Can you work these out from the model? Positions are in its coordinate system, mm. A direction names the side the tool comes from. Give positions to 0.01 mm unless a question says otherwise; leave off trailing zeros. Order: outer loops, then holes, each group sorted by start corner. A loop starts at its lowest first (then second) coordinate and runs counter-clockwise, first axis right, second up. Notation, with made-up numbers: M 19,-22 L 24,-22 A15 ccw 24,-7 Z; hole C -2.5,76 d6. An arc over 180 degrees is marked long. Answer as a JSON object with one key per item and string values.
```python
from build123d import *

# Parameters (mm, degrees)
SKETCH1_W           = 52
SKETCH1_H           = 24
SKETCH1_R           = 8.25
BOSS_EXTRUDE1_DEPTH = 12
SKETCH2_R           = 1
CUT_EXTRUDE1_DEPTH  = 32.048349393
SKETCH3_R           = 1.75
CUT_EXTRUDE2_DEPTH  = 1
FILLET1_R           = 2.5
CUT_EXTRUDE3_DEPTH  = 5
FILLET2_R           = 0.5
SKETCH6_W           = 10
SKETCH6_H           = 10
SKETCH6_R           = 2
BOSS_EXTRUDE2_DEPTH = 5
FILLET3_R           = 4.6
FILLET4_R           = 3


with BuildPart() as part:
    # Sketch1 → Boss-Extrude1 (new body)
    with BuildSketch(Plane(origin=(0, 0, 0), x_dir=(1, 0, 0), z_dir=(0, 1, 0))):
        Rectangle(SKETCH1_W, SKETCH1_H)
        with Locations(Location((12.75, 0, 0), (0, 0, 270))):
            Circle(SKETCH1_R, mode=Mode.SUBTRACT)
        with Locations(Location((-12.75, 0, 0), (0, 0, 270))):
            Circle(SKETCH1_R, mode=Mode.SUBTRACT)
    extrude(amount=BOSS_EXTRUDE1_DEPTH)

    # Sketch2 → Cut-Extrude1 (cut, through all)
    with BuildSketch(Plane(origin=(0, 12, 0), x_dir=(1, 0, 0), z_dir=(0, 1, 0))):
        with Locations(Location((-21.35, 8.85, 0), (0, 0, 270))):
            Circle(SKETCH2_R)
        with Locations(Location((21.35, 8.85, 0), (0, 0, 270))):
            Circle(SKETCH2_R)
        with Locations(Location((21.35, -8.85, 0), (0, 0, 270))):
            Circle(SKETCH2_R)
        with Locations(Location((-21.35, -8.85, 0), (0, 0, 270))):
            Circle(SKETCH2_R)
    extrude(amount=-CUT_EXTRUDE1_DEPTH, mode=Mode.SUBTRACT)

    # Sketch3 → Cut-Extrude2 (cut)
    with BuildSketch(Plane(origin=(0, 12, 0), x_dir=(1, 0, 0), z_dir=(0, 1, 0))):
        with Locations(Location((-21.35, 8.85, 0), (0, 0, 270))):
            Circle(SKETCH3_R)
        with Locations(Location((21.35, 8.85, 0), (0, 0, 270))):
            Circle(SKETCH3_R)
        with Locations(Location((21.35, -8.85, 0), (0, 0, 270))):
            Circle(SKETCH3_R)
        with Locations(Location((-21.35, -8.85, 0), (0, 0, 270))):
            Circle(SKETCH3_R)
    extrude(amount=-CUT_EXTRUDE2_DEPTH, mode=Mode.SUBTRACT)

    # Fillet1
    fillet1_edges = [part.edges().sort_by_distance(p)[0] for p in [
        (26, 6, 12),
        (-26, 6, 12),
        (-26, 6, -12),
        (26, 6, -12),
    ]]
    fillet(fillet1_edges, radius=FILLET1_R)

    # Sketch4 → Cut-Extrude3 (cut)
    with BuildSketch(Plane.XZ):
        Polygon((-6, -5), (-6, -12), (6, -12), (6, -5), (0, -5), align=None)
    extrude(amount=-CUT_EXTRUDE3_DEPTH, mode=Mode.SUBTRACT)

    # Fillet2
    fillet2_edges = [part.edges().sort_by_distance(p)[0] for p in [
        (0, 5, -12),
        (6, 2.5, -12),
        (-6, 2.5, -12),
        (-6, 2.5, -5),
        (6, 5, -8.5),
        (6, 2.5, -5),
        (-6, 5, -8.5),
        (0, 5, -5),
    ]]
    fillet(fillet2_edges, radius=FILLET2_R)

    # Sketch6 → Boss-Extrude2 (add)
    # profile 1 of 2: a face of its own
    with BuildSketch(Plane(origin=(0, 12, 0), x_dir=(1, 0, 0), z_dir=(0, 1, 0))):
        with Locations((-31, 0)):
            Rectangle(SKETCH6_W, SKETCH6_H)
        with Locations(Location((-31, 0, 0), (0, 0, 270))):
            Circle(SKETCH6_R, mode=Mode.SUBTRACT)
    # profile 2 of 2: a face of its own
    with BuildSketch(Plane(origin=(0, 12, 0), x_dir=(1, 0, 0), z_dir=(0, 1, 0))):
        with Locations((31, 0)):
            Rectangle(SKETCH6_W, SKETCH6_H)
        with Locations(Location((31, 0, 0), (0, 0, 90))):
            Circle(SKETCH6_R, mode=Mode.SUBTRACT)
    extrude(amount=-BOSS_EXTRUDE2_DEPTH)

    # Fillet3
    # the kernel refuses this fillet: 4.6 mm, written as the material it adds along each edge
    with BuildSketch(Plane(origin=(26, 12, 5), x_dir=(-5.467859312132584e-05, 0, 0.9999999985051258), z_dir=(0, -1, 0)), Plane(origin=(-26, 12, -5), x_dir=(5.467859312132586e-05, 0, -0.9999999985051258), z_dir=(0, -1, 0))) as fillet3_piece_1:
        with BuildLine():
            CenterArc((4.59974851, -4.599547254), FILLET3_R, 90.80387664, 89.192990507)
            Line((-0.000251483, -4.599295733), (-0.460251482, -4.599270581))
            Line((-0.460251482, -4.599270581), (-0.459999999, 2.5152e-05))
            Line((-0.459999999, 2.5152e-05), (2.5152e-05, 0.459999999))
            ThreePointArc((2.5152e-05, 0.459999999), (4.500025145, 0.459753946), (4.528757551, 0.459954725))
            Line((4.528757551, 0.459954725), (4.535211274, 0))
        make_face()
    extrude(amount=5)
    with BuildSketch(Plane(origin=(-26, 12, 5), x_dir=(5.467859312289258e-05, 0, 0.9999999985051258), z_dir=(0, -1, 0)), Plane(origin=(26, 12, -5), x_dir=(-5.467859312132581e-05, 0, -0.9999999985051258), z_dir=(0, -1, 0))) as fillet3_piece_2:
        with BuildLine():
            CenterArc((4.59974851, 4.599547254), FILLET3_R, 180.003132853, 89.192990507)
            Line((-0.000251483, 4.599295733), (-0.460251482, 4.599270581))
            Line((-0.460251482, 4.599270581), (-0.459999999, -2.5152e-05))
            Line((-0.459999999, -2.5152e-05), (2.5152e-05, -0.459999999))
            ThreePointArc((2.5152e-05, -0.459999999), (4.500025145, -0.459753946), (4.528757551, -0.459954725))
            Line((4.528757551, -0.459954725), (4.535211274, 0))
        make_face()
    extrude(amount=5)

    # Fillet4
    fillet4_edges = [part.edges().sort_by_distance(p)[0] for p in [
        (-36, 9.5, 5),
        (-36, 9.5, -5),
        (36, 9.5, -5),
        (36, 9.5, 5),
    ]]
    fillet(fillet4_edges, radius=FILLET4_R)


solid = part.part
```
1) Thinking about a two-plate mould opening in Z: for faces 4 (the face through (27.405, 9.535, -6.289)), 5 (the face through (-20.36, 5.58, 8.72)), 6 (the face through (-25.287, 6.084, 11.248)), 7 (the face through (4.7, 5.9, -1.8)), which applies, pulls with the +Z half, pulls with the -Z half, needs draft (parallel to the pull), parting line crosses it, or undercut?
Results found:
{"face 4": "pulls with the -Z half", "face 5": "undercut", "face 6": "pulls with the +Z half", "face 7": "undercut"}
2) I want a section at B-B on y = 2. Write out the boundary of the cut face in (x, z).
Results found:
{"outline": "M -26,-9.5 A2.5 ccw -23.5,-12 L -6.5,-12 A0.5 ccw -6,-11.5 L -6,-5.5 A0.5 cw -5.5,-5 L 5.5,-5 A0.5 cw 6,-5.5 L 6,-11.5 A0.5 ccw 6.5,-12 L 23.5,-12 A2.5 ccw 26,-9.5 L 26,9.5 A2.5 ccw 23.5,12 L -23.5,12 A2.5 ccw -26,9.5 Z; hole C -21.35,-8.85 d2; hole C -21.35,8.85 d2; hole C -12.75,0 d16.5; hole C 12.75,0 d16.5; hole C 21.35,-8.85 d2; hole C 21.35,8.85 d2"}
3) I need wall thicknesses on L1, parallel to X at y = 10.35, z = 0; L2, parallel to X at y = 3, z = 9; L3, parallel to X at y = 4.25, z = 0. Which ranges of each line are inside material? Lowest first, please.
Results found:
{"L1": "x = -36 to -33, -29 to -21, -4.5 to 4.5, 21 to 29, 33 to 36", "L2": "x = -26 to -22.34, -20.36 to 20.36, 22.34 to 26", "L3": "x = -26 to -21, -4.5 to 4.5, 21 to 26"}
4) I'm going to push flat-ended pins straight in: pin 1 Ø1 at (x, z) = (21.5, 8.5) entering from +Y; pin 2 Ø3.5 at (y, z) = (3.5, 4.5) entering from -X; pin 3 Ø3 at (x, z) = (-1, -7) entering from -Y; pin 4 Ø1.2 at (x, y) = (32, 10.5) entering from -Z. Where does each tip first touch, or does it pass through?
Results found:
{"pin 1": "passes through", "pin 2": "stops at x = -26", "pin 3": "stops at y = 5", "pin 4": "stops at z = -5"}
5) For faces 1 (the face through (-26, 3, 0)), 2 (the face through (-6, 2, -8)), 3 (the face through (-23.06, 11.51, 8.47)), which set-ups out of +Z, -Z, +X, -X, +Y, -Y let a thin tool reach every point of the face, with its end or its side?
Results found:
{"face 1": "+Z, -Z, -X, -Y", "face 2": "-Z, -Y", "face 3": "+Y"}
6) I want a section at A-A on z = 0. Write out the boundary of the cut face in (x, y).
Results found:
{"outline": "M -36,7 L -33,7 L -33,12 L -36,12 Z; M -29,7 L -26,7 L -26,0 L -21,0 L -21,12 L -29,12 Z; M -4.5,0 L 4.5,0 L 4.5,12 L -4.5,12 Z; M 21,0 L 26,0 L 26,7 L 29,7 L 29,12 L 21,12 Z; M 33,7 L 36,7 L 36,12 L 33,12 Z"}
7) I want a section at D-D on y = 8.5. Count the separate pieces of the cut face and the enclosed holes in it, and give its area (3 significant figures).
Results found:
{"separate pieces": "1", "enclosed holes": "8", "area": "988 mm²"}
8) I want a section at C-C on x = -18.5. Write out the boundary of the cut face in (y, z), and give its area (3 significant figures).
Results found:
{"outline": "M 0,-12 L 12,-12 L 12,-5.92 L 0,-5.92 Z; M 0,5.92 L 12,5.92 L 12,12 L 0,12 Z", "area": "146 mm²"}
